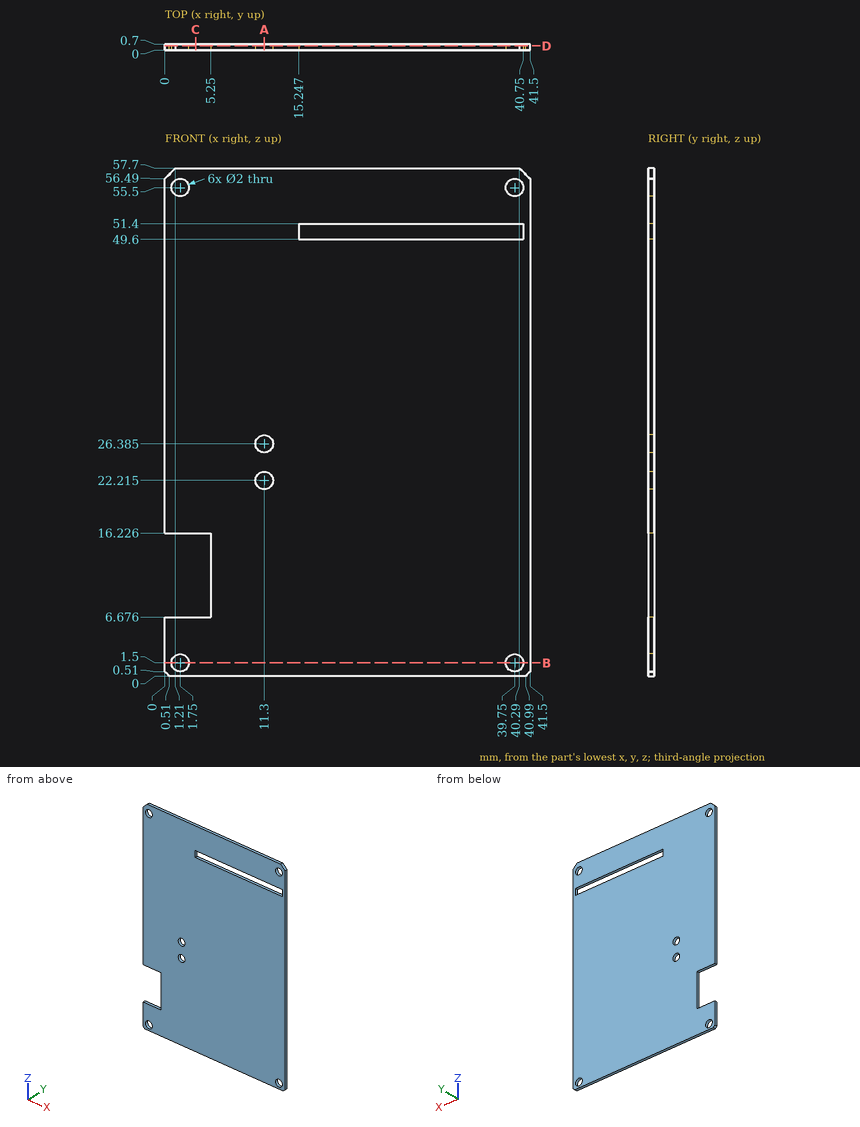
Study the drawing (mm; zero at the part's minimum x, y, z) and answer. Give positions to 0.01 mm unless a question says otherwise; leave off trailing zeros. Order: outer loops, then holes, each group sorted by start corner. A loop starts at its lowest first (then second) coordinate and runs counter-clockwise, first axis right, second up. Notation, with made-up numbers: (-37.5, -15) -> (20.5, -15) arc R18 cw to (20.5, 20) -> close; hole circle Ø1 at (89.25, 51). An arc over 180 degrees is marked (long way). Put each result on its own line as item: value.
Item 1: A cutting plane is placed at C-C on x = 3.5. Give the vertices of the cut face in (y, z).
Established:
outline: (0, 0) -> (0.7, 0) -> (0.7, 6.68) -> (0, 6.68) -> close; (0, 16.23) -> (0.7, 16.23) -> (0.7, 57.7) -> (0, 57.7) -> close
Item 2: Straight lines are drawn through the part: line 1 (Z direction, x = 1.75, y = 0.2); line 2 (X direction, y = 0.45, z = 1.5); line 3 (Z direction, x = 39.75, y = 0.4). For each, find the intervals that lie inside material, in ascending order.
Established:
line 1: z = 0 to 0.5, 2.5 to 6.68, 16.23 to 54.5, 56.5 to 57.7
line 2: x = 0 to 0.75, 2.75 to 38.75, 40.75 to 41.5
line 3: z = 0 to 0.5, 2.5 to 49.6, 51.4 to 54.5, 56.5 to 57.7
Item 3: A cutting plane is placed at D-D on y = 0.5. Count the separate pieces of the cut face and the enclosed holes in it, plus the area to 3 significant figures.
Established:
separate pieces: 1
enclosed holes: 7
area: 2,280 mm^2
Item 4: A cutting plane is placed at B-B on z = 1.5. Give the vertices of the cut face in (x, y).
Established:
outline: (0, 0) -> (0.75, 0) -> (0.75, 0.7) -> (0, 0.7) -> close; (2.75, 0) -> (38.75, 0) -> (38.75, 0.7) -> (2.75, 0.7) -> close; (40.75, 0) -> (41.5, 0) -> (41.5, 0.7) -> (40.75, 0.7) -> close
Item 5: Given P1, Ø3, axis at x = 34, z = 44.5, coming from the -Y side, flat-ended and moving along its own axis, determine where the tip first touches the part or whether it passes through.
Established:
P1: stops at y = 0
Item 6: A cutting plane is placed at A-A on x = 11.3. Give the vertices of the cut face in (y, z) (1 decimal).
Established:
outline: (0, 0) -> (0.7, 0) -> (0.7, 21.2) -> (0, 21.2) -> close; (0, 23.2) -> (0.7, 23.2) -> (0.7, 25.4) -> (0, 25.4) -> close; (0, 27.4) -> (0.7, 27.4) -> (0.7, 57.7) -> (0, 57.7) -> close
